from build123d import *

# Parameters (mm, degrees)
EXTRUDE_1_DEPTH   = 2
HOLE_WIZARD_M81_D = 9
CHAMFER_1_SIZE    = 2.5


with BuildPart() as part:
    # Эскиз3 → Бобышка-Вытянуть1 (new body)
    with BuildSketch(Plane(origin=(0, 0, 0), x_dir=(1, 0, 0), z_dir=(0, 0, -1))):
        Polygon((0, 0), (90, 0), (90, 113.431457505), (61.715728753, 141.715728753), (0, 80), align=None)
    extrude(amount=EXTRUDE_1_DEPTH)

    # Отверстие с зазором M81 (through all)
    with Locations(Plane(origin=(0, 0, -2), x_dir=(1, 0, 0), z_dir=(0, 0, -1))):
        with Locations((20, 20), (70, 20), (28.284271247, 80), (61.715728753, 113.431457505)):
            Hole(HOLE_WIZARD_M81_D / 2)

    # Фаска1
    chamfer_1_edges = [part.edges().sort_by_distance(p)[0] for p in [
        (61.715728753, -141.715728753, -1),
        (90, 0, -1),
        (0, 0, -1),
    ]]
    chamfer(chamfer_1_edges, length=CHAMFER_1_SIZE)


solid = part.part
Model file for the job. Use its own axes, mm. Give positions to 0.01 mm unless a question says otherwise; leave off trailing zeros. Order: outer loops, then holes, each group sorted by start corner. A loop starts at its lowest first (then second) coordinate and runs counter-clockwise, first axis right, second up. Notation, with made-up numbers: (-33.5, -15.75) - (25.5, -15.75) arc R22 cw to (25.5, 20.25) - close; hole circle Ø3 at (81, 56). An arc over 180 degrees is marked (long way). Write item = value, one per line. Start each with the question number.
1. Cut at B-B, the plane z = -1.55. List the corners of the cut face in (x, y).
2. Cut at A-A, the plane y = -20. List the corners of the cut face in (x, z).
3. Cut at C-C, the plane x = 20. List the corners of the cut face in (y, z).
4. Drop a flat-ended pin along its axis: P1, Ø7, axis at x = 61.72, y = -113.43, coming from the +Z side. Give the stop position or say it passes through.
5. Cut at D-D, the plane x = 43. List the corners of the cut face in (y, z).
6. Probe line 1 along X through (y, z) = (-20, -1.3); line 2 along X through (y, z) = (-80, -0.5); line 3 along Y through (x, z) = (19.5, -1.2). List the from-to ranges inside material, lowest first.
7. Two-plate mould, pull along X, no slides. Class faces 1 (the flat face through (88.8, -1.3, -1)), 2 (the flat face through (30, -110, -1)), 3 (the cylindrical face through (67.581, -23.794, -0.986)), 4 (the cylindrical face through (28.87, -84.46, -0.99)): pulls with the +X half, pulls with the -X half, needs draft (parallel to the pull), parting line crosses it, or undercut.
Taken from the geometry:
q1.outline = (0, -80) - (59.95, -139.95) - (63.48, -139.95) - (90, -113.43) - (90, -2.5) - (87.5, 0) - (2.5, 0) - (0, -2.5) - close; hole circle Ø9 at (20, -20); hole circle Ø9 at (28.28, -80); hole circle Ø9 at (61.72, -113.43); hole circle Ø9 at (70, -20)
q2.outline = (0, -2) - (15.5, -2) - (15.5, 0) - (0, 0) - close; (24.5, -2) - (65.5, -2) - (65.5, 0) - (24.5, 0) - close; (74.5, -2) - (90, -2) - (90, 0) - (74.5, 0) - close
q3.outline = (-100, -2) - (-24.5, -2) - (-24.5, 0) - (-100, 0) - close; (-15.5, -2) - (0, -2) - (0, 0) - (-15.5, 0) - close
q4.P1 = through
q5.outline = (-123, -2) - (0, -2) - (0, 0) - (-123, 0) - close
q6.line_1 = 0 to 15.5, 24.5 to 65.5, 74.5 to 90
q6.line_2 = 0 to 23.78, 32.78 to 90
q6.line_3 = -99.5 to -24.47, -15.53 to 0
q7.face_1 = pulls with the +X half
q7.face_2 = pulls with the -X half
q7.face_3 = undercut
q7.face_4 = undercut
